Design review of the part built by this model. Coordinates are the model's own, in mm. A direction names the side the tool comes from. Round coordinates to 2 decimals unless told otherwise and drop trailing zeros. Write each loop counter-clockwise with the first axis right and the second up, starting at its lowest first coordinate (ties: lowest second). Pieces come first, ordered by that corner, then holes. Notation, with made-up numbers: M 84.5,37.5 L 89.5,37.5 A27 ccw 89.5,76.5 Z; hole C -38,67 d11. An arc over 180 degrees is marked long. One line per question, with ' | ' between items. Start each with the question number.
Item 1: For L1, parallel to Z at x = 57, y = 65.5; L2, parallel to X at y = 121, z = 28; L3, parallel to Y at x = -63, z = -20, list the stretches that pass through material, from the lowest coordinate up.
Item 2: Add section D-D, the plane z = -29. State the section outline as (x, y) points.
Item 3: Add section C-C, the plane x = -6. State the section outline as (y, z) points, and give its area (3 significant figures).
Item 4: Insertion check: pin 1 Ø3 at (x, z) = (73, -46.5) entering from -Y; pin 2 Ø6 at (x, z) = (-22, 39.5) entering from -Y; pin 3 Ø12 at (x, z) = (4.5, 17.5) entering from +Y; pin 4 Ø18 at (x, z) = (-51, 3) entering from -Y. Each pin has a flat end and moves straight along its axis. Give the tip position at first contact, or say it passes through.
Item 5: Machinability: for faces 1 (the face through (-57, 36, 0)), 2 (the face through (-73, 3, -47)), 3 (the face through (-54, 17, 18.06)), which of the approach directions +Z, -Z, +X, -X, +Y, -Y give a long, thin tool a straight path to every point of the face, cutting with its end or side? Answer none if there is none.
Item 6: Add section B-B, the plane y = 99. State the section outline as (x, z) points, and give its area (3 significant figures).
Item 7: Draft analysis for pull direction Z (two halves, no side actions). For faces 4 (the face through (73, 3, -47)), 5 (the face through (-76.129, 74, -1)), state which applies: released by +Z, released by -Z, zero draft, split by the parting line, or undercut.
Item 8: Add section A-A, the plane z = 4. State the section outline as (x, y) points.
```python
from build123d import *

# Parameters (mm, degrees)
BOSS_EXTRUDE7_DEPTH  = 150
SKETCH2_42_R         = 2
CUT_EXTRUDE8_DEPTH   = 3
SHELL4_DEPTH         = 148
SHELL4_START         = 5
SHELL4_2_DEPTH       = 143
SKETCH2_43_W         = 45.023033392
SKETCH2_43_H         = 36
BOSS_EXTRUDE8_DEPTH  = 36
SKETCH2_44_W         = 45.023033392
SKETCH2_44_H         = 36
CUT_EXTRUDE9_DEPTH   = 33
CUT_EXTRUDE11_DEPTH  = 33
FILLET4_R            = 1
BOSS_EXTRUDE11_DEPTH = 40
CUT_EXTRUDE16_DEPTH  = 40


# Read off the part's stored shape, not the designer's step: Shell4
with BuildPart() as part:
    # Sketch2 → Boss-Extrude7 (new body)
    with BuildSketch(Plane(origin=(0, 0, 0), x_dir=(1, 0, 0), z_dir=(0, 1, 0))):
        with BuildLine():
            Line((-76.129191463, 48.939688446), (-76.129191463, -49.060311554))
            ThreePointArc((-76.129191463, -49.060311554), (-75.836298244, -49.767418335), (-75.129191463, -50.060311554))
            Line((-75.129191463, -50.060311554), (74.870808537, -50.060311554))
            ThreePointArc((74.870808537, -50.060311554), (75.577915319, -49.767418335), (75.870808537, -49.060311554))
            Line((75.870808537, -49.060311554), (75.870808537, 48.939688446))
            ThreePointArc((75.870808537, 48.939688446), (75.577915319, 49.646795227), (74.870808537, 49.939688446))
            Line((74.870808537, 49.939688446), (-75.129191463, 49.939688446))
            ThreePointArc((-75.129191463, 49.939688446), (-75.836298244, 49.646795227), (-76.129191463, 48.939688446))
        make_face()
    extrude(amount=BOSS_EXTRUDE7_DEPTH)

    # Sketch2<42> → Cut-Extrude8 (cut)
    with BuildSketch(Plane(origin=(0, 0, 0), x_dir=(1, 0, 0), z_dir=(0, 1, 0))):
        with Locations(Location((-73.129191463, 46.939688446, 0), (0, 0, 270))):
            Circle(SKETCH2_42_R)
        with Locations(Location((72.870808537, 46.939688446, 0), (0, 0, 270))):
            Circle(SKETCH2_42_R)
        with Locations(Location((72.870808537, -47.060311554, 0), (0, 0, 270))):
            Circle(SKETCH2_42_R)
        with Locations(Location((-73.129191463, -47.060311554, 0), (0, 0, 270))):
            Circle(SKETCH2_42_R)
    extrude(amount=CUT_EXTRUDE8_DEPTH, mode=Mode.SUBTRACT)

    # Shell4 outline → Shell4 (cut)
    with BuildSketch(Plane(origin=(0, 0, 0), x_dir=(1, 0, 0), z_dir=(0, 1, 0))):
        with BuildLine():
            Line((-74.129191463, 43.0667051), (-74.129191463, -43.187328208))
            ThreePointArc((-74.129191463, -43.187328208), (-70.300764338, -44.231884429), (-69.256208116, -48.060311554))
            Line((-69.256208116, -48.060311554), (68.997825191, -48.060311554))
            ThreePointArc((68.997825191, -48.060311554), (70.042381413, -44.231884429), (73.870808537, -43.187328208))
            Line((73.870808537, -43.187328208), (73.870808537, 43.0667051))
            ThreePointArc((73.870808537, 43.0667051), (70.042381413, 44.111261321), (68.997825191, 47.939688446))
            Line((68.997825191, 47.939688446), (-69.256208116, 47.939688446))
            ThreePointArc((-69.256208116, 47.939688446), (-70.300764338, 44.111261321), (-74.129191463, 43.0667051))
        make_face()
    extrude(amount=SHELL4_DEPTH, mode=Mode.SUBTRACT)

    # Shell4 2 outline → Shell4 2 (cut)
    with BuildSketch(Plane(origin=(0, 0, 0), x_dir=(1, 0, 0), z_dir=(0, 1, 0)).offset(SHELL4_START)):
        with BuildLine():
            Line((-74.129191463, -43.187328208), (-74.129191463, -48.060311554))
            Line((-74.129191463, -48.060311554), (-69.256208116, -48.060311554))
            ThreePointArc((-69.256208116, -48.060311554), (-70.300764338, -44.231884429), (-74.129191463, -43.187328208))
        make_face()
        with BuildLine():
            Line((-74.129191463, 47.939688446), (-74.129191463, 43.0667051))
            ThreePointArc((-74.129191463, 43.0667051), (-70.300764338, 44.111261321), (-69.256208116, 47.939688446))
            Line((-69.256208116, 47.939688446), (-74.129191463, 47.939688446))
        make_face()
        with BuildLine():
            ThreePointArc((73.870808537, -43.187328208), (70.042381413, -44.231884429), (68.997825191, -48.060311554))
            Line((68.997825191, -48.060311554), (73.870808537, -48.060311554))
            Line((73.870808537, -48.060311554), (73.870808537, -43.187328208))
        make_face()
        with BuildLine():
            Line((73.870808537, 47.939688446), (68.997825191, 47.939688446))
            ThreePointArc((68.997825191, 47.939688446), (70.042381413, 44.111261321), (73.870808537, 43.0667051))
            Line((73.870808537, 43.0667051), (73.870808537, 47.939688446))
        make_face()
    extrude(amount=SHELL4_2_DEPTH, mode=Mode.SUBTRACT)

    # Sketch2<43> → Boss-Extrude8 (add)
    with BuildSketch(Plane(origin=(0, 0, 0), x_dir=(1, 0, 0), z_dir=(0, 1, 0))):
        Polygon((-76.129191463, -20.060311554), (-29.106158071, -20.060311554), (-29.106158071, 19.939688446), (-76.129191463, 19.939688446), (-76.129191463, 17.939688446), (-31.106158071, 17.939688446), (-31.106158071, -18.060311554), (-76.129191463, -18.060311554), align=None)
        with Locations((-53.617674767, -0.060311554)):
            Rectangle(SKETCH2_43_W, SKETCH2_43_H)
    extrude(amount=BOSS_EXTRUDE8_DEPTH)

    # Sketch2<44> → Cut-Extrude9 (cut)
    with BuildSketch(Plane(origin=(0, 0, 0), x_dir=(1, 0, 0), z_dir=(0, 1, 0))):
        with Locations((-53.617674767, -0.060311554)):
            Rectangle(SKETCH2_44_W, SKETCH2_44_H)
    extrude(amount=CUT_EXTRUDE9_DEPTH, mode=Mode.SUBTRACT)

    # Sketch7 → Cut-Extrude11 (cut)
    with BuildSketch(Plane.XZ.offset(-33)):
        with BuildLine():
            Line((-49.385393046, -8.706663468), (-49.385393046, 8.706663468))
            ThreePointArc((-49.385393046, 8.706663468), (-42.00713359, 16.084922924), (-34.628874134, 8.706663468))
            Line((-34.628874134, 8.706663468), (-34.628874134, -8.706663468))
            ThreePointArc((-34.628874134, -8.706663468), (-42.00713359, -16.084922924), (-49.385393046, -8.706663468))
        make_face()
    extrude(amount=-CUT_EXTRUDE11_DEPTH, mode=Mode.SUBTRACT)

    # Fillet4
    fillet4_edges = [part.edges().sort_by_distance(p)[0] for p in [
        (-76.129191463, 33, 0.060311554),
    ]]
    fillet(fillet4_edges, radius=FILLET4_R)

    # Sketch8 → Boss-Extrude11 (add)
    with BuildSketch(Plane(origin=(0, 150, 0), x_dir=(1, 0, 0), z_dir=(0, 1, 0))):
        with BuildLine():
            Line((2.680111603, -13.646632902), (2.680111603, 13.646632902))
            ThreePointArc((2.680111603, 13.646632902), (12.409959802, 23.376481102), (22.139808002, 13.646632902))
            Line((22.139808002, 13.646632902), (22.139808002, -13.646632902))
            ThreePointArc((22.139808002, -13.646632902), (12.409959802, -23.376481102), (2.680111603, -13.646632902))
        make_face()
    extrude(amount=-BOSS_EXTRUDE11_DEPTH)

    # Sketch8<7> → Cut-Extrude16 (cut)
    with BuildSketch(Plane(origin=(0, 150, 0), x_dir=(1, 0, 0), z_dir=(0, 1, 0))):
        with BuildLine():
            Line((2.680111603, -13.646632902), (2.680111603, 13.646632902))
            ThreePointArc((2.680111603, 13.646632902), (12.409959802, 23.376481102), (22.139808002, 13.646632902))
            Line((22.139808002, 13.646632902), (22.139808002, -13.646632902))
            ThreePointArc((22.139808002, -13.646632902), (12.409959802, -23.376481102), (2.680111603, -13.646632902))
        make_face()
    extrude(amount=-CUT_EXTRUDE16_DEPTH, mode=Mode.SUBTRACT)


solid = part.part
```
Computed values:
1) L1: z = -49.94 to -47.94, 48.06 to 50.06 | L2: x = -76.13 to -74.13, 73.87 to 75.87 | L3: y = 148 to 150
2) outline: M -76.13,0 L -74.13,0 L -74.13,148 L 73.87,148 L 73.87,0 L 75.87,0 L 75.87,150 L -76.13,150 Z
3) outline: M 0,-49.94 L 150,-49.94 L 150,50.06 L 0,50.06 L 0,48.06 L 148,48.06 L 148,-47.94 L 0,-47.94 Z | area: 792 mm^2
4) pin 1: stops at y = 3 | pin 2: stops at y = 148 | pin 3: stops at y = 150 | pin 4: stops at y = 33
5) face 1: none | face 2: -Y | face 3: -X, -Y
6) outline: M -76.13,-48.94 A1 ccw -75.13,-49.94 L 74.87,-49.94 A1 ccw 75.87,-48.94 L 75.87,49.06 A1 ccw 74.87,50.06 L -75.13,50.06 A1 ccw -76.13,49.06 Z; hole M -74.13,-47.94 L 73.87,-47.94 L 73.87,48.06 L -74.13,48.06 Z | area: 991 mm^2
7) face 4: undercut | face 5: zero draft
8) outline: M -76.13,34 A1 ccw -75.13,33 L -49.39,33 L -49.39,36 L -74.13,36 L -74.13,148 L 2.68,148 L 2.68,150 L -76.13,150 Z; M -34.63,33 L -31.11,33 L -31.11,0 L -29.11,0 L -29.11,36 L -34.63,36 Z; M 22.14,148 L 73.87,148 L 73.87,0 L 75.87,0 L 75.87,150 L 22.14,150 Z
